Autodesk Inventor part; units mm, degrees
ref_plane "YZ Plane" through (0, 0, 0) normal (1, 0, 0) x (0, 1, 0)
ref_plane "XZ Plane" through (0, 0, 0) normal (0, 1, 0) x (-1, 0, 0)
ref_plane "XY Plane" through (0, 0, 0) normal (0, 0, 1) x (1, 0, 0)
sketch "スケッチ1" plane through (0, 0, 0) normal (0, 0, 1) x (1, 0, 0)
  line L0 (0, 0) -> (10, 0)
  line L1 (10, 0) -> (10, -10)
  line L2 (10, -10) -> (0, -10)
  line L3 (0, -10) -> (0, 0)
  line L4 (0, -5) -> (10, -5)
  line L5 (5, 0) -> (5, -10)
  dimension "d0" = 10
  dimension "d1" = 10
extrude "押し出し1" add sketch "スケッチ1" along normal blind 10
sketch "スケッチ2" plane through (10, -10, 0) normal (1, 0, 0) x (0, 0, -1)
  line L0 (-10, 10) -> (0, 10)
  line L1 (0, 10) -> (0, 0)
  line L2 (0, 0) -> (-10, 0)
  line L3 (-10, 0) -> (-10, 10)
  line L4 (-10, 10) -> (0, 0)
  line L5 (0, 10) -> (0, 0)
  line L6 (-10, 0) -> (0, 10)
  point P0 (-5, 5)
hole "穴1" at (10, -5, 5) direction (-1, 0, 0) diameter 2.5 end through all
sketch "スケッチ3" plane through (0, 0, 0) normal (0, 1, 0) x (1, 0, 0)
  line L0 (10, 0) -> (10, -10)
  line L1 (10, -10) -> (0, -10)
  line L2 (0, -10) -> (0, 0)
  line L3 (0, 0) -> (10, 0)
  line L4 (0, -10) -> (10, 0)
  line L5 (10, 0) -> (10, -10)
  line L6 (0, 0) -> (10, 0)
  line L7 (10, -10) -> (0, 0)
  point P0 (5, -5)
hole "穴2" at (5, 0, 5) direction (0, -1, 0) diameter 2.5 end through all
properties part number "垂直ブロック 樹脂 10" material "PPS プラスチック"
Verification items for the finished model (mm, model axes). Coordinates: 2 decimals unless noted, no trailing zeros. Order: outer loops, then holes, each group sorted by start corner. A loop starts at its lowest first (then second) coordinate and runs counter-clockwise, first axis right, second up. Notation, with made-up numbers: (25.5, 84) -> (65.5, 84) arc R25 ccw to (65.5, 100) -> close; hole circle Ø2 at (47, -22.75). An arc over 180 degrees is marked (long way). Use CSV: the item, a comma, the result in double quotes. Start each with the question number.
Q1. Draft check along Y on faces 1 (the flat face through (5, -5, 0)), 2 (the cylindrical face through (1.91, -5.05, 6.25)), 3 (the flat face through (6, -10, 4)). Enter one of: +Y half, -Y half, draft (parallel to the pull), parting line (faces both ways), or undercut.
Q2. Section check A-A, the plane x = 6. Record the cut outline in (y, z), and give its area (3 significant figures).
Q3. Section check C-C, the plane x = 1.25. Record the cut outline in (y, z).
Q4. Section check D-D, the plane y = -9. Record the cut outline in (x, z).
Q5. Thickness scan on line 1 along X through (y, z) = (-6.45, 5); line 2 along Y through (x, z) = (3.1, 5). Record the ranges inside material, lowest first.
Q6. Section check B-B, the plane z = 5. Record the cut outline in (x, y).
Returned:
1,face 1,"draft"
1,face 2,"undercut"
1,face 3,"-Y half"
2,outline,"(-10, 0) -> (0, 0) -> (0, 4.25) -> (-4, 4.25) arc R1.25 cw to (-6, 4.25) -> (-10, 4.25) -> close; (-10, 5.75) -> (-6, 5.75) arc R1.25 cw to (-4, 5.75) -> (0, 5.75) -> (0, 10) -> (-10, 10) -> close"
2,area,"83.6 mm^2"
3,outline,"(-10, 0) -> (0, 0) -> (0, 10) -> (-10, 10) -> close; hole circle Ø2.5 at (-5, 5)"
4,outline,"(0, 0) -> (10, 0) -> (10, 10) -> (0, 10) -> close; hole circle Ø2.5 at (5, 5)"
5,line 1,"x = 0 to 3.75, 6.25 to 10"
5,line 2,"y = -10 to -6.25, -3.75 to 0"
6,outline,"(0, -10) -> (3.75, -10) -> (3.75, -6.25) -> (0, -6.25) -> close; (0, -3.75) -> (3.75, -3.75) -> (3.75, 0) -> (0, 0) -> close; (6.25, -10) -> (10, -10) -> (10, -6.25) -> (6.25, -6.25) -> close; (6.25, -3.75) -> (10, -3.75) -> (10, 0) -> (6.25, 0) -> close"
